Source: CAD feature listing. Evaluate the final solid. Frame: model axes, mm. Coordinates: 2 decimals unless noted, no trailing zeros. Write each loop counter-clockwise with the first axis right and the second up, starting at its lowest first coordinate (ties: lowest second). Pieces come first, ordered by that corner, then holes. Notation, with made-up numbers: M 54,6.5 L 93,6.5 A26 ccw 93,38.5 Z; hole C 50.25,30 d1. An arc over 180 degrees is marked long. Write item = value, one per line. Start each with the question number.
1. Line query: line 1 along Y through (x, z) = (0, 64); line 2 along X through (y, z) = (2.5, 77.5); line 3 along X through (y, z) = (1.25, 19). Output: solid intervals per line, ascending.
2. Pin query (flat end, axial travel): pin 1 Ø8 at (x, z) = (0, 61.5) entering from -Y; pin 2 Ø5 at (y, z) = (-1.5, 40.5) entering from -X; pin 3 Ø2 at (y, z) = (-4, 49.5) entering from -X. Return the tip coordinate at first contact, or that it passes through.
3. Section query A-A (z = 19). Output: boundary loops of the cut face in (x, y), then the cut area to 3 significant figures.
4. Section query B-B (y = -5.75). Output: boundary loops of the cut face in (x, z).
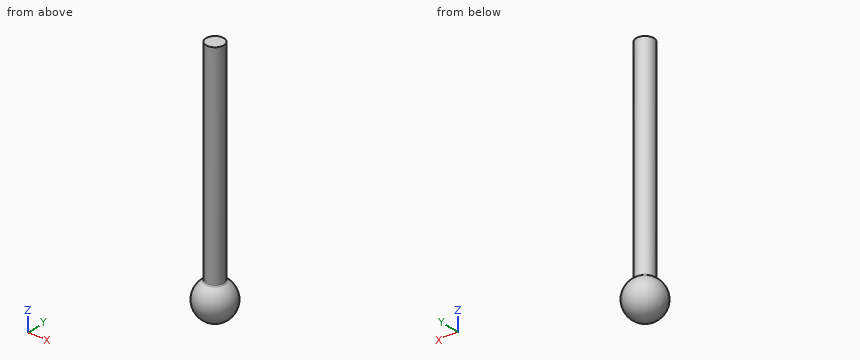
```python
from build123d import *

# Parameters (mm, degrees)
ESBO_O1_R                = 3.5
RESSALTO_EXTRUS_O1_DEPTH = 85
FILETE1_R                = 0.5


with BuildPart() as part:
    # Esboço1 → Ressalto-extrusão1 (new body)
    with BuildSketch(Plane.XY):
        Circle(ESBO_O1_R)
    extrude(amount=RESSALTO_EXTRUS_O1_DEPTH)

    # Esboço2 → Revolução7 (revolve)
    with BuildSketch(Plane(origin=(0, 0, 0), x_dir=(1, 0, 0), z_dir=(0, 1, 0))):
        with BuildLine():
            Line((0, 13), (0, -2))
            ThreePointArc((0, -2), (-7.5, 5.5), (0, 13))
        make_face()
    revolve(axis=Axis((0, 0, -13), (0, 0, 1)))

    # Filete1
    filete1_edges = [part.edges().sort_by_distance(p)[0] for p in [
        (0, 3.5, 1.133249581),
    ]]
    fillet(filete1_edges, radius=FILETE1_R)


solid = part.part
```
Results are:
q1.line_1 = -3.5 to 3.5
q1.line_2 = -2.45 to 2.45
q1.line_3 = -3.27 to 3.27
q2.pin_1 = -3.5
q2.pin_2 = -3.5
q2.pin_3 = -1.8
q3.outline = C 0,0 d7
q3.area = 38.5 mm^2
q4.outline = C 0,-5.5 d9.63
